from build123d import *

# Parameters (mm, degrees)
F1_DEPTH = 20
F3_DEPTH = 15
F4_R     = 5
F4_R_2   = 7.5
F5_DEPTH = 5
F7_R     = 6
F8_DEPTH = 45


with BuildPart() as f1:
    # F0 (on Front) → F1 (new body)
    with BuildSketch(Plane.XZ):
        with BuildLine():
            ThreePointArc((2.666667, 15.776213), (-16, 0), (2.666667, -15.776213))
            Line((2.666667, -15.776213), (20.166667, -12.818173))
            ThreePointArc((20.166667, -12.818173), (31, 0), (20.166667, 12.818173))
            Line((20.166667, 12.818173), (2.666667, 15.776213))
        make_face()
    extrude(amount=F1_DEPTH)

    # F2 (on face) → F3 (cut)
    with BuildSketch(Plane.XZ.offset(20)):
        with BuildLine():
            Line((19.666667, 9.860133), (2.166667, 12.818173))
            ThreePointArc((2.166667, 12.818173), (-13, 0), (2.166667, -12.818173))
            Line((2.166667, -12.818173), (19.666667, -9.860133))
            ThreePointArc((19.666667, -9.860133), (28, 0), (19.666667, 9.860133))
        make_face()
    extrude(amount=-F3_DEPTH, mode=Mode.SUBTRACT)

    # F4 (on face) → F5 (cut)
    with BuildSketch(Plane.XZ.offset(5)):
        with Locations((18, 0)):
            Circle(F4_R)
        Circle(F4_R_2)
    extrude(amount=-F5_DEPTH, mode=Mode.SUBTRACT)

    # F7 (on offset) → F8 (join)
    with BuildSketch(Plane.YZ.offset(30)):
        with Locations((-10, 0)):
            Circle(F7_R)
    extrude(amount=F8_DEPTH)


solid = f1.part
The model under review builds one solid part; all positions refer to its coordinate system, in mm. A direction names the side the tool comes from. Round coordinates to 2 decimals unless told otherwise and drop trailing zeros. Loops run counter-clockwise (first coordinate to the right, second up) from the corner with the lowest first, then second, coordinate; pieces in that order, holes last. Notation, with made-up numbers: (-3.5, -37.75) -> (52.5, -37.75) arc R29 cw to (52.5, -13.75) -> close; hole circle Ø10 at (8, 14.25). An arc over 180 degrees is marked (long way). Return JSON: item names as keys, results as strings.
(1) For faces 4 (the cylindrical face through (52.185, -4.277, 1.802)), 5 (the flat face through (11.04, -12.6, 11.32)), 6 (the cylindrical face through (13, -3, 0)), list the 3-axis set-ups (+Z, -Z, +X, -X, +Y, -Y) from which the entire face can be reached by the end or side of a thin tool; tool diameter is ignored.
Solved:
{"face 4": "+X", "face 5": "-Y", "face 6": "+Y, -Y"}
(2) For line 1 (Z direction, x = 0, y = -3.8); line 2 (Z direction, x = 0, y = -12.5); line 3 (X direction, y = -2.5, z = 6), list the stretches that pass through material, from the lowest coordinate up.
Solved:
{"line 1": "-16 to -7.5, 7.5 to 16", "line 2": "-16 to -13, 13 to 16", "line 3": "-14.83 to -4.5, 4.5 to 29.53"}
(3) For pin 1 (8 mm diameter, centred on x = 22.5, y = -10.5, fed in from -Z); pin 2 (0.8 mm diameter, centred on y = -8.5, z = 5.5, fed in from -X); pin 3 (6 mm diameter, centred on x = -6.5, y = -3.5, fed in from +Z); pin 4 (8 mm diameter, centred on x = 64, z = 10.5, fed in from -Y), all flat-tipped, find the tip position at first contact; note any pin that passes through.
Solved:
{"pin 1": "z = -13.1", "pin 2": "x = -15.17", "pin 3": "z = 15.61", "pin 4": "through"}
(4) Add section B-B on x = 0. Write out the cut boundary in (y, z), plus the area to 3 significant figures.
Solved:
{"outline": "(-20, -16) -> (0, -16) -> (0, -7.5) -> (-5, -7.5) -> (-5, -13) -> (-20, -13) -> close; (-20, 13) -> (-5, 13) -> (-5, 7.5) -> (0, 7.5) -> (0, 16) -> (-20, 16) -> close", "area": "175 mm2"}
(5) Add section D-D on y = -17.5. Write out the cut boundary in (x, z), plus the area to 3 significant figures.
Solved:
{"outline": "(2.67, -15.78) -> (20.17, -12.82) arc R13 ccw to (20.17, 12.82) -> (2.67, 15.78) arc R16 ccw (long way) to start; hole (2.17, -12.82) -> (19.67, -9.86) arc R10 ccw to (19.67, 9.86) -> (2.17, 12.82) arc R13 ccw (long way) to start", "area": "355 mm2"}
(6) Add section A-A on z = 0. Write out the cut boundary in (x, y), plus the area to 3 significant figures.
Solved:
{"outline": "(-16, -20) -> (-13, -20) -> (-13, -5) -> (-7.5, -5) -> (-7.5, 0) -> (-16, 0) -> close; (7.5, -5) -> (13, -5) -> (13, 0) -> (7.5, 0) -> close; (23, -5) -> (28, -5) -> (28, -20) -> (31, -20) -> (31, -16) -> (75, -16) -> (75, -4) -> (31, -4) -> (31, 0) -> (23, 0) -> close", "area": "728 mm2"}
(7) Add section C-C on y = -1. Write out the cut boundary in (x, z).
Solved:
{"outline": "(2.67, -15.78) -> (20.17, -12.82) arc R13 ccw to (20.17, 12.82) -> (2.67, 15.78) arc R16 ccw (long way) to start; hole circle Ø15 at (0, 0); hole circle Ø10 at (18, 0)"}
(8) The part is to be moulded in two halves that separate along Z. For faces 1 (the flat face through (7.2, 0, -3.3)), 2 (the cylindrical face through (-16, -10, 0)), 3 (the flat face through (7.2, -5, 3.1)), say which applies: released by +Z, released by -Z, zero draft, split by the parting line, or undercut.
Solved:
{"face 1": "zero draft", "face 2": "split by the parting line", "face 3": "undercut"}
